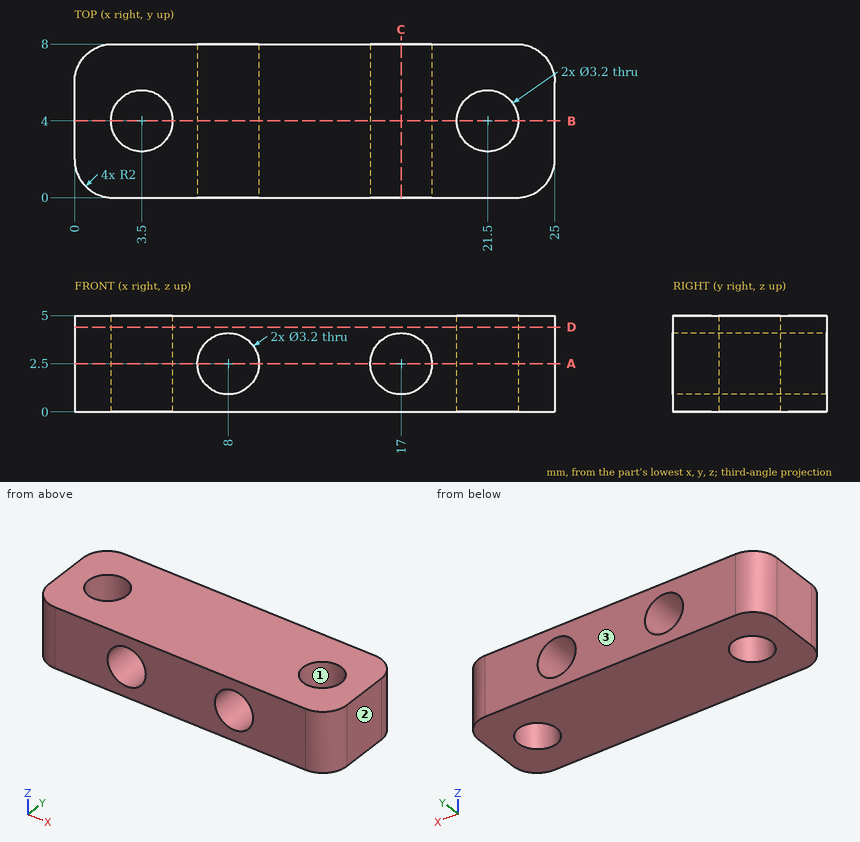
Here's the drawing with two shaded views (mm, measured from the low corner). I have some questions. Coordinates: 2 decimals unless noted, no trailing zeros. Write each loop counter-clockwise with the first axis right and the second up, starting at its lowest first coordinate (ties: lowest second). Pieces come first, ordered by that corner, then holes.
Item 1: I want a section at A-A on z = 2.5. Write out the boundary of the cut face in (x, y), and give its area (3 significant figures).
Item 2: I want a section at D-D on z = 4.4. Write out the boundary of the cut face in (x, y), and give its area (3 significant figures).
Item 3: I want a section at C-C on x = 17. Write out the boundary of the cut face in (y, z).
Item 4: If we mould it in two halves opening along Y, with no side actions, what happens to the marked faces 1, 2 and 3? For each: +Y half, -Y half, draft (parallel to the pull), parting line (faces both ways), or undercut.
Item 5: If I drill on line 1 (Y direction, x = 3.5, z = 3.15); line 2 (X direction, y = 2.25, z = 1.25); line 3 (X direction, y = 1.25, z = 1.65), over which ranges is the centre line in solid material (lowest first)?
Item 6: I want a section at B-B on y = 4. Write out the boundary of the cut face in (x, z).
Item 7: Will this pin go through, and if not, where does the flat tip stop? pin 1 (4 mm diameter, centred on x = 21.5, y = 4, fed in from -Z).
Findings below:
1. outline: (0, 2) arc R2 ccw to (2, 0) - (6.4, 0) - (6.4, 8) - (2, 8) arc R2 ccw to (0, 6) - close; (9.6, 0) - (15.4, 0) - (15.4, 8) - (9.6, 8) - close; (18.6, 0) - (23, 0) arc R2 ccw to (25, 2) - (25, 6) arc R2 ccw to (23, 8) - (18.6, 8) - close; hole circle Ø3.2 at (3.5, 4); hole circle Ø3.2 at (21.5, 4)
1. area: 129 mm2
2. outline: (0, 2) arc R2 ccw to (2, 0) - (23, 0) arc R2 ccw to (25, 2) - (25, 6) arc R2 ccw to (23, 8) - (2, 8) arc R2 ccw to (0, 6) - close; hole circle Ø3.2 at (3.5, 4); hole circle Ø3.2 at (21.5, 4)
2. area: 180 mm2
3. outline: (0, 0) - (8, 0) - (8, 0.9) - (0, 0.9) - close; (0, 4.1) - (8, 4.1) - (8, 5) - (0, 5) - close
4. face 1: undercut
4. face 2: draft
4. face 3: +Y half
5. line 1: y = 0 to 2.4, 5.6 to 8
5. line 2: x = 0 to 7, 9 to 16, 18 to 25
5. line 3: x = 0.15 to 6.64, 9.36 to 15.64, 18.36 to 24.85
6. outline: (0, 0) - (1.9, 0) - (1.9, 5) - (0, 5) - close; (5.1, 0) - (19.9, 0) - (19.9, 5) - (5.1, 5) - close; (23.1, 0) - (25, 0) - (25, 5) - (23.1, 5) - close; hole circle Ø3.2 at (8, 2.5); hole circle Ø3.2 at (17, 2.5)
7. pin 1: stops at z = 0
